```python
from build123d import *

# Parameters (mm, degrees)
F0_W     = 2
F0_H     = 15.5
F0_W_2   = 125
F1_DEPTH = 2.5
F2_DEPTH = 6


with BuildPart() as f1:
    # F0 (on Top) → F1 (new body)
    with BuildSketch(Plane.XY):
        with Locations((63.5, 0)):
            Rectangle(F0_W, F0_H)
        Rectangle(F0_W_2, F0_H)
        with Locations((-63.5, 0)):
            Rectangle(F0_W, F0_H)
    extrude(amount=F1_DEPTH)

    # F0 (on Top) → F2 (join)
    with BuildSketch(Plane.XY):
        with Locations((-63.5, 0)):
            Rectangle(F0_W, F0_H)
        with Locations((63.5, 0)):
            Rectangle(F0_W, F0_H)
    extrude(amount=-F2_DEPTH)


solid = f1.part
```
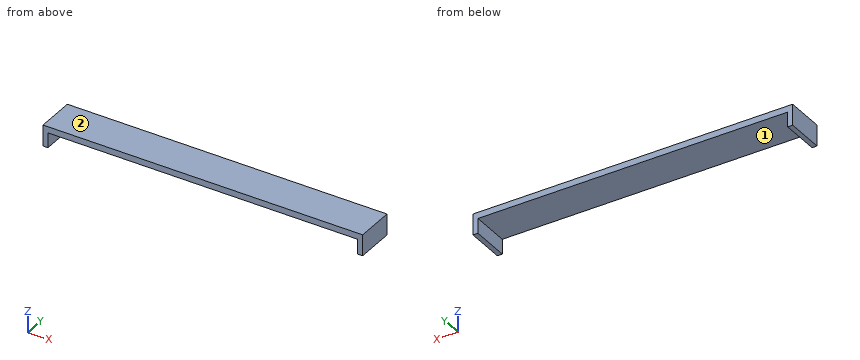
Here's how the part is built. I have some questions about the finished solid (model axes, mm). Face numbers are marked on the shaded views. Coordinates: 2 decimals unless noted, no trailing zeros. Loops run counter-clockwise (first coordinate to the right, second up) from the corner with the lowest first, then second, coordinate; pieces in that order, holes last. Notation, with made-up numbers: (79, 20) - (135, 20) arc R32 ccw to (135, 56) - close; hole circle Ø2 at (-8, 17). An arc over 180 degrees is marked (long way). Answer as CSV lines item,"result".
Q1. If we section it at B-B, the plane y = 3: Write out the boundary of the cut face in (x, z), and give its area (4 significant figures).
Response:
outline,"(-64.5, -6) - (-62.5, -6) - (-62.5, 0) - (62.5, 0) - (62.5, -6) - (64.5, -6) - (64.5, 2.5) - (-64.5, 2.5) - close"
area,"346.5 mm2"
Q2. If we section it at C-C, the plane x = -38: Write out the boundary of the cut face in (y, z), and give its area (4 significant figures).
Response:
outline,"(-7.75, 0) - (7.75, 0) - (7.75, 2.5) - (-7.75, 2.5) - close"
area,"38.75 mm2"
Q3. If I drill on L1, parallel to X at y = -0.25, z = -3.5; L2, parallel to Z at x = -14.5, y = -0.5, over which ranges is the centre line in solid material (lowest first)? Write a range as [from, to].
Response:
L1,"[-64.5, -62.5], [62.5, 64.5]"
L2,"[0, 2.5]"
Q4. For pin 1 (4.5 mm diameter, centred on x = -5, y = -3.5, fed in from -Z), with a flat end and sliding along its axis, tell me the tip position at first contact or that it passes through.
Response:
pin 1,"z = 0"
Q5. If we section it at A-A, the plane z = -4.25: Write out the boundary of the cut face in (x, y).
Response:
outline,"(-64.5, -7.75) - (-62.5, -7.75) - (-62.5, 7.75) - (-64.5, 7.75) - close; (62.5, -7.75) - (64.5, -7.75) - (64.5, 7.75) - (62.5, 7.75) - close"
Q6. We'd pull the mould along X, two halves only. Please class the marked faces 1 and 2: pulls with the +X half, pulls with the -X half, needs draft (parallel to the pull), parting line crosses it, or undercut.
Response:
face 1,"undercut"
face 2,"needs draft"
